The listing builds one solid part. Answer for the finished solid, in the listing's coordinates (mm). A direction names the side the tool comes from. Give positions to 0.01 mm unless a question says otherwise; leave off trailing zeros. Write each loop counter-clockwise with the first axis right and the second up, starting at its lowest first coordinate (ties: lowest second). Pieces come first, ordered by that corner, then holes. Notation, with made-up numbers: (37, 56) - (55, 56) arc R31 ccw to (55, 93) - close; hole circle Ø6 at (48, 79). An arc over 180 degrees is marked (long way). One line per question, with ' | ' between items. Start each with the question number.
1. For faces 1 (the face through (7, 2, 12)), 2 (the face through (-472.129, 30.518, 0.986)), determine the directions among +Z, -Z, +X, -X, +Y, -Y from which every point of the face is accessible in a straight line to the end or side of a thin tool.
2. Given P1, Ø5, axis at x = 99.5, z = 10.5, coming from the +Y side; P2, Ø1.5, axis at x = -111, y = 22, coming from the +Z side; P3, Ø1, axis at y = 39.5, z = 1, coming from the -X side, each flat-ended and moving along its own axis, determine where each tip first touches the part or whether it passes through.
3. A cutting plane is placed at B-B (z = 13.5). Determine the outline of the cut face in (x, y).
4. Find the intervals of material crossed by L1, parallel to Z at x = -119.5, y = 4; L2, parallel to Z at x = 362.5, y = 17, in increasing order. Write a range as from..to.
5. A cutting plane is placed at A-A (x = 0). Determine the outline of the cut face in (y, z).
6. A cutting plane is placed at D-D (x = -126). Determine the outline of the cut face in (y, z).
Autodesk Inventor part; units mm, degrees
ref_plane "YZ Plane" through (0, 0, 0) normal (1, 0, 0) x (0, 1, 0)
ref_plane "XZ Plane" through (0, 0, 0) normal (0, 1, 0) x (-1, 0, 0)
ref_plane "XY Plane" through (0, 0, 0) normal (0, 0, 1) x (1, 0, 0)
sketch "Sketch1" plane through (0, 0, 0) normal (0, 0, 1) x (1, 0, 0)
  line L0 (-490, 48) -> (490, 48)
  line L1 (490, 48) -> (490, 0)
  line L2 (490, 0) -> (-490, 0)
  line L3 (-490, 0) -> (-490, 48)
  point P0 (0, 0)
  point P1 (0, 0)
  dimension "d0" = 980
  dimension "d1" = 48
extrude "Plate1" add sketch "Sketch1" along normal blind 2
sketch "Sketch2" plane through (490, 2, 0) normal (0, -1, 0) x (1, 0, 0)
  line L0 (-980, 0) -> (0, 0)
  line L1 (0, 0) -> (0, 20)
  line L2 (0, 20) -> (-980, 20)
  line L3 (-980, 20) -> (-980, 0)
edge flange "Flange1" height 20 angle 90 thickness 2 bend radius 2.75 thickness toward (0, -1, 0) relief round relief width 2 relief depth 1 edges at (0, 0, 2) wall of the first edge with corners at (-490, 2, 0) (490, 2, 0) (490, 2, 20) (-490, 2, 20)
bend "Bend1"
corner "Corner1"
sketch "Sketch5" plane through (0, 0, 0) normal (0, 0, -1) x (-1, 0, 0)
  line L0 (490, 48) -> (-490, 48)
  line L1 (490, 0) -> (-490, 0)
  circle A0 centre (0, 48) radius 25
  line L2 (243.95, 48) -> (246.05, 48)
  line L3 (246.05, 48) -> (246.05, 27)
  line L4 (246.05, 27) -> (243.95, 27)
  line L5 (243.95, 27) -> (243.95, 48)
  line L6 (-243.95, 48) -> (-246.05, 48)
  line L7 (-246.05, 48) -> (-246.05, 27)
  line L8 (-246.05, 27) -> (-243.95, 27)
  line L9 (-243.95, 27) -> (-243.95, 48)
  line L10 (0, 48) -> (0, 0) construction
  line L11 (490, 0) -> (490, 48)
  line L12 (-490, 0) -> (-490, 48)
  circle A1 centre (-490, 48) radius 25
  circle A2 centre (490, 48) radius 25
  point P0 (0, 0)
  point P1 (245, 27)
  point P2 (-245, 27)
  point P3 (246.05, 48)
  point P4 (-25, 48)
  point P5 (25, 48)
  point P6 (-246.05, 48)
  point P7 (465, 48)
  point P8 (490, 23)
  point P9 (-490, 23)
  point P10 (-465, 48)
  dimension "d45" = 50
  dimension "d48" = 2.1
  dimension "d49" = 490
  dimension "d51" = 27
  dimension "d52" = 21
extrude "Extrusion1" cut sketch "Sketch5" against normal through all contours L3 L4 L5 L0 | L0 L11 A2 | A0 L0 | L9 L8 L7 L0 picked at (473.5423, 46.1457) picked at (-2.955, 40.2082)
sketch "Sketch9" plane through (0, 0, 2) normal (0, 0, 1) x (1, 0, 0)
  line L0 (480.2878, 24.3045) -> (480.2878, 12.3045) construction
  line L1 (480.2878, 12.3045) -> (280.2878, 12.3045) construction
  line L2 (280.2878, 12.3045) -> (280.2878, 24.3045) construction
  line L3 (280.2878, 24.3045) -> (480.2878, 24.3045) construction
  line L4 (-490, 48) -> (490, 48)
  point P0 (0, 0)
  point P1 (1.05, 68)
  point P2 (490, 48)
  point P3 (-490, 48)
  dimension "d40" = 200
  dimension "d41" = 12
mark "Mark2"
equation "\"d2\" = Thickness"
equation "\"d3\" = BendReliefWidth"
equation "\"d4\" = BendReliefDepth"
equation "\"d5\" = MinimumRemnant"
equation "\"d6\" = TransitionRadius"
equation "\"d9\" = BendRadius"
equation "\"d10\" = CornerReliefSize"
equation "\"d11\" = GapSize"
equation "\"d12\" = JacobiRadiusSize"
equation "\"BendReliefWidth\" = Thickness"
equation "\"BendReliefDepth\" = 0.5 * Thickness"
equation "\"CornerReliefSize\" = 4 * Thickness"
equation "\"MinimumRemnant\" = 2 * Thickness"
equation "\"TransitionRadius\" = BendRadius"
equation "\"JacobiRadiusSize\" = BendRadius"
equation "\"GapSize\" = Thickness"
properties part number "MSC 325 STRINGER BOARD  ##" material "Stainless Steel"
Determined:
1) face 1: +Z, +X, -X, +Y | face 2: +Z, -Z, -X, +Y
2) P1: y = 2 | P2: z = 2 | P3: x = -466.68
3) outline: (-490, 0) - (490, 0) - (490, 2) - (-490, 2) - close
4) L1: 0.06..2.1 | L2: 0..2
5) outline: (0, 4.75) arc R4.75 ccw to (4.75, 0) - (23, 0) - (23, 2) - (4.75, 2) arc R2.75 cw to (2, 4.75) - (2, 20) - (0, 20) - close
6) outline: (0, 4.75) arc R4.75 ccw to (4.75, 0) - (48, 0) - (48, 2) - (4.75, 2) arc R2.75 cw to (2, 4.75) - (2, 20) - (0, 20) - close
